Check sheet for the modelled part. Datum: model origin and axes. Units: mm. Face numbers are marked on the shaded views. A direction names the side the tool comes from. Give positions to 0.01 mm unless a question says otherwise; leave off trailing zeros. Write each loop counter-clockwise with the first axis right and the second up, starting at its lowest first coordinate (ties: lowest second). Pieces come first, ordered by that corner, then holes.
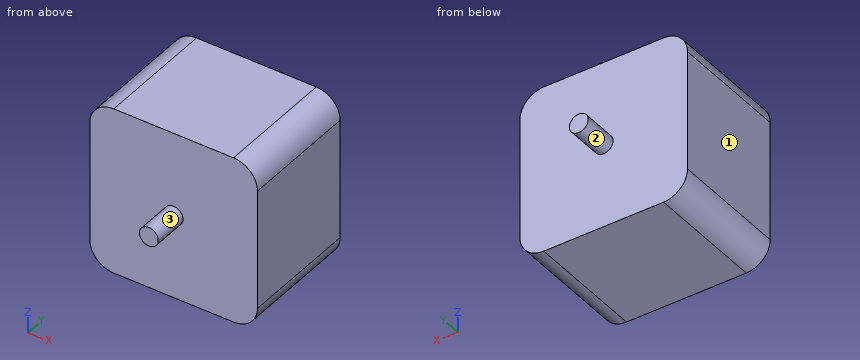
from build123d import *

# Parameters (mm, degrees)
SKETCH1_W           = 44.45
SKETCH1_H           = 44.45
BOSS_EXTRUDE1_DEPTH = 31.75
FILLET1_R           = 6.35
SKETCH2_R           = 2.5
BOSS_EXTRUDE2_DEPTH = 9.525
SKETCH4_R           = 2.5
BOSS_EXTRUDE3_DEPTH = 9.525


with BuildPart() as part:
    # Sketch1 → Boss-Extrude1 (new body)
    with BuildSketch(Plane(origin=(0, 0, 0), x_dir=(1, 0, 0), z_dir=(0, 1, 0))):
        Rectangle(SKETCH1_W, SKETCH1_H)
    extrude(amount=BOSS_EXTRUDE1_DEPTH)

    # Fillet1
    fillet1_edges = [part.edges().sort_by_distance(p)[0] for p in [
        (22.225, 15.875, 22.225),
        (-22.225, 15.875, 22.225),
        (-22.225, 15.875, -22.225),
        (22.225, 15.875, -22.225),
    ]]
    fillet(fillet1_edges, radius=FILLET1_R)

    # Sketch2 → Boss-Extrude2 (add)
    with BuildSketch(Plane(origin=(0, 31.75, 0), x_dir=(1, 0, 0), z_dir=(0, 1, 0))):
        Circle(SKETCH2_R)
    extrude(amount=BOSS_EXTRUDE2_DEPTH)

    # Sketch4 → Boss-Extrude3 (add)
    with BuildSketch(Plane.XZ):
        Circle(SKETCH4_R)
    extrude(amount=BOSS_EXTRUDE3_DEPTH)


solid = part.part
1) Sectioned sample at A-A on x = 0. Record the boundary of the cut face in (y, z) (3 decimals), then the cut area to 3 significant figures.
2) Sectioned sample at C-C on z = -1.5. Record the boundary of the cut face in (x, y) (3 decimals).
3) Scan lines: L1, parallel to X at y = 32.5, z = 0; L2, parallel to Y at x = -13, z = -9; L3, parallel to X at y = 19, z = 16. Record each from-to range of solid material in increasing order.
4) Access from +Z, -Z, +X, -X, +Y, -Y to the whole of each face (thin tool, end or side, straight path). Record for the marked faces 1, 2 and 3.
5) Gauge pin test, flat ends, axial feed: pin 1 (2 mm diameter, centred on x = 16.5, z = 0.5, fed in from -Y); pin 2 (2 mm diameter, centred on x = 16, z = 3.5, fed in from +Y). Record the tip position at first contact, or that the pin passes through.
6) Sectioned sample at D-D on x = 11.5. Record the boundary of the cut face in (y, z) (3 decimals), then the cut area to 3 significant figures.
7) Sectioned sample at B-B on y = 15. Record the boundary of the cut face in (x, z) (3 decimals).
Answers below:
1. outline: (-9.525, -2.5) - (0, -2.5) - (0, -22.225) - (31.75, -22.225) - (31.75, -2.5) - (41.275, -2.5) - (41.275, 2.5) - (31.75, 2.5) - (31.75, 22.225) - (0, 22.225) - (0, 2.5) - (-9.525, 2.5) - close
1. area: 1,510 mm2
2. outline: (-22.225, 0) - (-2, 0) - (-2, -9.525) - (2, -9.525) - (2, 0) - (22.225, 0) - (22.225, 31.75) - (2, 31.75) - (2, 41.275) - (-2, 41.275) - (-2, 31.75) - (-22.225, 31.75) - close
3. L1: x = -2.5 to 2.5
3. L2: y = 0 to 31.75
3. L3: x = -22.22 to 22.22
4. face 1: +Z, -Z, -X, +Y, -Y
4. face 2: +Y
4. face 3: -Y
5. pin 1: stops at y = 0
5. pin 2: stops at y = 31.75
6. outline: (0, -22.225) - (31.75, -22.225) - (31.75, 22.225) - (0, 22.225) - close
6. area: 1,410 mm2
7. outline: (-22.225, -15.875) arc R6.35 ccw to (-15.875, -22.225) - (15.875, -22.225) arc R6.35 ccw to (22.225, -15.875) - (22.225, 15.875) arc R6.35 ccw to (15.875, 22.225) - (-15.875, 22.225) arc R6.35 ccw to (-22.225, 15.875) - close
